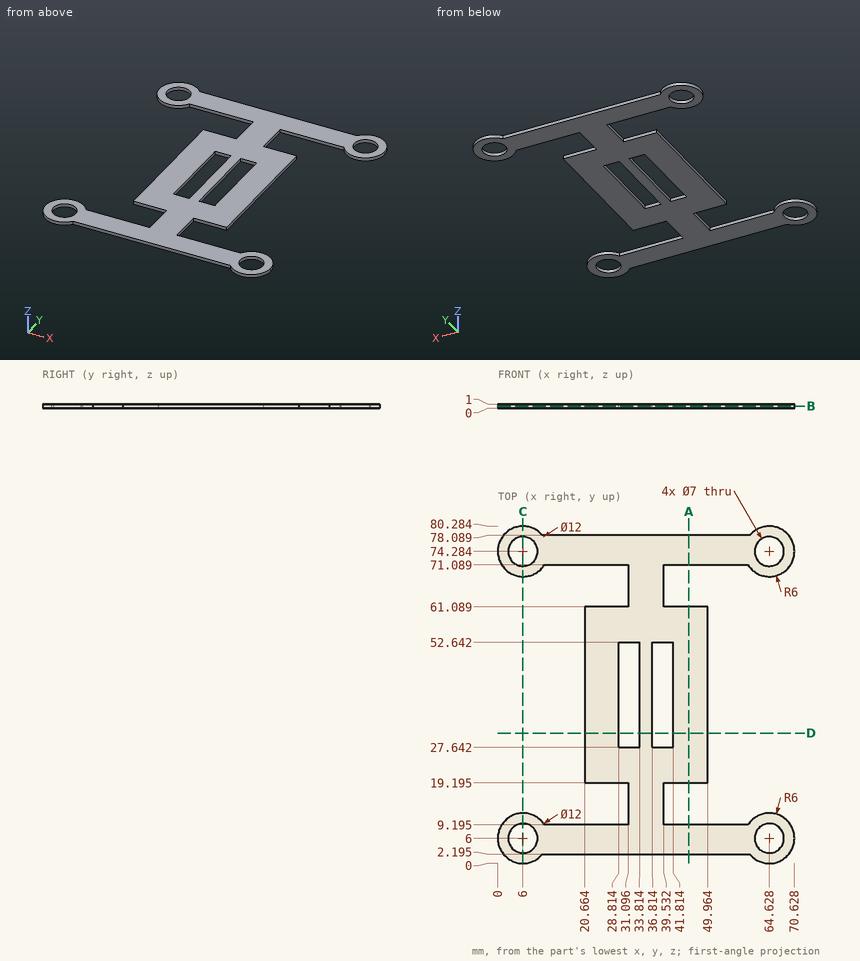
Input: dimensioned drawing with shaded views. Units: mm. Origin: part minimum x, y, z. Give positions to 0.01 mm unless a question says otherwise; leave off trailing zeros. Loops run counter-clockwise (first coordinate to the right, second up) from the corner with the lowest first, then second, coordinate; pieces in that order, holes last. Notation, with made-up numbers: (-39, 2.25) -> (4, 2.25) arc R13 ccw to (4, 19.25) -> close; hole circle Ø9 at (24, 6). An arc over 180 degrees is marked (long way). Use a Markdown table: item, result. Add a question column.
1) Section query C-C, the plane x = 6. Return the cut outline in (y, z) (1 decimal).
2) First-contact query: pin 1 (0.5 mm diameter, centred on y = 15.5, z = 0.5, fed in from -X); pin 2 (0.5 mm diameter, centred on y = 34.5, z = 0.5, fed in from -X); pin 3 (0.5 mm diameter, centred on x = 31.5, z = 0.5, fed in from +Y). Flat tips, straight axial feed; report the tip coordinate or a pass-through.
3) Section query B-B, the plane z = 0.5. Count the separate pieces of the cut face and the enclosed holes in it, then the cut area to 3 significant figures.
4) Line query: line 1 along Y through (x, z) = (6, 0.7) (1 decimal); line 2 along X through (y, z) = (40, 0.95) (1 decimal); line 3 along Y through (x, z) = (24.5, 0.4) (1 decimal). Output: solid intervals per line, ascending. Write a range as [from, to].
5) Section query A-A, the plane x = 45.5. Return the cut outline in (y, z) (1 decimal).
6) Section query D-D, the plane y = 31. Return the cut outline in (x, z) (1 decimal), then the cut area to 3 significant figures.
Numbers:
| question | item | result |
|---|---|---|
| 1 | outline | (0, 0) -> (2.5, 0) -> (2.5, 1) -> (0, 1) -> close; (9.5, 0) -> (12, 0) -> (12, 1) -> (9.5, 1) -> close; (68.3, 0) -> (70.8, 0) -> (70.8, 1) -> (68.3, 1) -> close; (77.8, 0) -> (80.3, 0) -> (80.3, 1) -> (77.8, 1) -> close |
| 2 | pin 1 | stops at x = 31.1 |
| 2 | pin 2 | stops at x = 20.66 |
| 2 | pin 3 | stops at y = 78.09 |
| 3 | separate pieces | 1 |
| 3 | enclosed holes | 6 |
| 3 | area | 2,110 mm2 |
| 4 | line 1 | y = [0, 2.5], [9.5, 12], [68.3, 70.8], [77.8, 80.3] |
| 4 | line 2 | x = [20.7, 28.8], [33.8, 36.8], [41.8, 50] |
| 4 | line 3 | y = [2.2, 9.2], [19.2, 61.1], [71.1, 78.1] |
| 5 | outline | (2.2, 0) -> (9.2, 0) -> (9.2, 1) -> (2.2, 1) -> close; (19.2, 0) -> (61.1, 0) -> (61.1, 1) -> (19.2, 1) -> close; (71.1, 0) -> (78.1, 0) -> (78.1, 1) -> (71.1, 1) -> close |
| 6 | outline | (20.7, 0) -> (28.8, 0) -> (28.8, 1) -> (20.7, 1) -> close; (33.8, 0) -> (36.8, 0) -> (36.8, 1) -> (33.8, 1) -> close; (41.8, 0) -> (50, 0) -> (50, 1) -> (41.8, 1) -> close |
| 6 | area | 19.3 mm2 |
